Geometry: final body of the model. Coordinates: model frame, mm. A direction names the side the tool comes from. Coordinates: 2 decimals unless noted, no trailing zeros. Write each loop counter-clockwise with the first axis right and the second up, starting at its lowest first coordinate (ties: lowest second). Pieces come first, ordered by that corner, then holes.
from build123d import *

# Parameters (mm, degrees)
ESQUISSE1_W             = 10
ESQUISSE1_H             = 10
BOSS_EXTRU_1_DEPTH      = 10
CONG_1_R                = 10
CONG_2_R                = 3
ESQUISSE2_R             = 1.8
ENL_V_MAT_EXTRU_1_DEPTH = 5
ESQUISSE3_R             = 1.8
ENL_V_MAT_EXTRU_2_DEPTH = 10
CONG_3_R                = 3


with BuildPart() as part:
    # Esquisse1 → Boss.-Extru.1 (new body)
    with BuildSketch(Plane.XY):
        Polygon((5, 29), (0, 29), (0, 0), (5, 0), (5, 14), (32.7, 14), (32.7, 6.5), (52.7, 6.5), (52.7, 14), (55.2, 14), (55.2, 0), (60.2, 0), (60.2, 29), (55.2, 29), (55.2, 21.5), (52.7, 21.5), (52.7, 26.5), (32.7, 26.5), (32.7, 21.5), (5, 21.5), align=None)
        with Locations((42.7, 16.5)):
            Rectangle(ESQUISSE1_W, ESQUISSE1_H, mode=Mode.SUBTRACT)
    extrude(amount=BOSS_EXTRU_1_DEPTH)

    # Congé1
    # the kernel refuses this fillet: 10 mm, written as the material it takes off along each edge
    with BuildSketch(Plane(origin=(52.7, 6.5, -24.206145914), x_dir=(-1, 0, 0), z_dir=(0, 0, 1))) as cong_1_piece_1:
        with BuildLine():
            CenterArc((9.682458366, -10), CONG_1_R, 90, 75.522487814)
            Line((0, -7.5), (-0.193649167, -7.45))
            ThreePointArc((-0.193649167, -7.45), (-0.2, -3.75), (-0.2, 0))
            Line((-0.2, 0), (0, 0.2))
            Line((0, 0.2), (9.682458366, 0.2))
            Line((9.682458366, 0.2), (9.682458366, 0))
        make_face()
    extrude(amount=58.412291828, mode=Mode.SUBTRACT)
    with BuildSketch(Plane(origin=(32.7, 6.5, -24.206145914), x_dir=(0, 1, 0), z_dir=(0, 0, 1))) as cong_1_piece_2:
        with BuildLine():
            CenterArc((10, -9.682458366), CONG_1_R, 104.477512186, 75.522487814)
            Line((0, -9.682458366), (-0.2, -9.682458366))
            Line((-0.2, -9.682458366), (-0.2, 0))
            Line((-0.2, 0), (0, 0.2))
            ThreePointArc((0, 0.2), (3.75, 0.2), (7.45, 0.193649167))
            Line((7.45, 0.193649167), (7.5, 0))
        make_face()
    extrude(amount=58.412291828, mode=Mode.SUBTRACT)
    with BuildSketch(Plane(origin=(52.7, 26.5, -21.650635095), x_dir=(0, -1, 0), z_dir=(0, 0, 1))) as cong_1_piece_3:
        with BuildLine():
            CenterArc((10, -8.660254038), CONG_1_R, 120, 60)
            Line((0, -8.660254038), (-0.2, -8.660254038))
            Line((-0.2, -8.660254038), (-0.2, 0))
            Line((-0.2, 0), (0, 0.2))
            ThreePointArc((0, 0.2), (2.5, 0.2), (4.9, 0.173205081))
            Line((4.9, 0.173205081), (5, 0))
        make_face()
    extrude(amount=53.301270189, mode=Mode.SUBTRACT)
    with BuildSketch(Plane(origin=(32.7, 26.5, -21.650635095), x_dir=(1, 0, 0), z_dir=(0, 0, 1))) as cong_1_piece_4:
        with BuildLine():
            CenterArc((8.660254038, -10), CONG_1_R, 90, 60)
            Line((0, -5), (-0.173205081, -4.9))
            ThreePointArc((-0.173205081, -4.9), (-0.2, -2.5), (-0.2, 0))
            Line((-0.2, 0), (0, 0.2))
            Line((0, 0.2), (8.660254038, 0.2))
            Line((8.660254038, 0.2), (8.660254038, 0))
        make_face()
    extrude(amount=53.301270189, mode=Mode.SUBTRACT)

    # Congé2
    cong_2_edges = [part.edges().sort_by_distance(p)[0] for p in [
        (47.7, 21.5, 5),
        (37.7, 21.5, 5),
        (37.7, 11.5, 5),
        (47.7, 11.5, 5),
    ]]
    fillet(cong_2_edges, radius=CONG_2_R)

    # Esquisse2 → Enlèv. mat.-Extru.1 (cut)
    with BuildSketch(Plane(origin=(60.2, 0, 0), x_dir=(0, 0, -1), z_dir=(1, 0, 0))):
        with Locations(Location((-5, 24, 0), (0, 0, 90))):
            Circle(ESQUISSE2_R)
        with Locations(Location((-5, 4, 0), (0, 0, 90))):
            Circle(ESQUISSE2_R)
    extrude(amount=-ENL_V_MAT_EXTRU_1_DEPTH, mode=Mode.SUBTRACT)

    # Esquisse3 → Enlèv. mat.-Extru.2 (cut)
    with BuildSketch(Plane.ZY):
        with Locations(Location((5, 25, 0), (0, 0, 270))):
            Circle(ESQUISSE3_R)
        with Locations(Location((5, 5, 0), (0, 0, 270))):
            Circle(ESQUISSE3_R)
    extrude(amount=-ENL_V_MAT_EXTRU_2_DEPTH, mode=Mode.SUBTRACT)

    # Congé3
    cong_3_edges = [part.edges().sort_by_distance(p)[0] for p in [
        (53.95, 14, 10),
        (57.7, 0, 10),
        (18.85, 14, 0),
        (2.5, 0, 0),
        (2.5, 29, 0),
        (57.7, 29, 10),
        (18.85, 21.5, 0),
        (53.95, 21.5, 0),
        (57.7, 29, 0),
        (57.7, 0, 0),
        (53.95, 14, 0),
        (53.95, 21.5, 10),
        (18.85, 21.5, 10),
        (2.5, 29, 10),
        (42.7, 6.5, 0),
        (42.7, 26.5, 0),
        (36.360254038, 25.160254038, 0),
        (49.039745962, 25.160254038, 0),
        (2.5, 0, 10),
        (36.258734009, 8.59430585, 0),
        (49.141265991, 8.59430585, 0),
        (42.7, 6.5, 10),
        (42.7, 26.5, 10),
        (36.360254038, 25.160254038, 10),
        (49.039745962, 25.160254038, 10),
        (36.258734009, 8.59430585, 10),
        (18.85, 14, 10),
        (49.141265991, 8.59430585, 10),
    ]]
    fillet(cong_3_edges, radius=CONG_3_R)


solid = part.part
Item 1: Pin query (flat end, axial travel): pin 1 (3 mm diameter, centred on x = 21.5, z = 6, fed in from -Y); pin 2 (5 mm diameter, centred on x = 20, z = 5, fed in from +Y); pin 3 (3 mm diameter, centred on x = 53.5, z = 4.5, fed in from +Y). Return the tip coordinate at first contact, or that it passes through.
Derived:
pin 1: stops at y = 14
pin 2: stops at y = 21.5
pin 3: stops at y = 22.55
Item 2: Pull-direction query (Z, two-part tool) for faces 6 (the cylindrical face through (2.465, 4.169, 3.403)), 7 (the cylindrical face through (57.74, 0.9, 0.86)), 8 (the cylindrical face through (36.424, 25.197, 4.972)); classes: released by +Z, released by -Z, zero draft, split by the parting line, or undercut.
Derived:
face 6: undercut
face 7: released by -Z
face 8: zero draft
Item 3: Section C-C, the plane y = 4. Output: boundary loops of the cut face in (x, z).
Derived:
outline: (0, 0) - (5, 0) - (5, 3.5) - (0, 3.5) - close; (0, 6.5) - (5, 6.5) - (5, 10) - (0, 10) - close; (55.2, 0) - (60.2, 0) - (60.2, 3.2) - (55.2, 3.2) - close; (55.2, 6.8) - (60.2, 6.8) - (60.2, 10) - (55.2, 10) - close
Item 4: Section A-A, the plane x = 31. Output: boundary loops of the cut face in (y, z).
Derived:
outline: (14, 3) arc R3 ccw to (17, 0) - (18.5, 0) arc R3 ccw to (21.5, 3) - (21.5, 7) arc R3 ccw to (18.5, 10) - (17, 10) arc R3 ccw to (14, 7) - close
Item 5: Material intervals for probe 1 along Z at (x, y) = (57.4, 24); probe 2 along X at (y, z) = (26.75, 3.25); probe 3 along X at (y, z) = (10.75, 2), sorted ascending.
Derived:
probe 1: z = 0 to 3.2, 6.8 to 10
probe 2: x = 0 to 5, 55.2 to 60.2
probe 3: x = 0 to 5, 34.41 to 50.99, 55.2 to 60.2
Item 6: Set-up query: faces 1 (the cylindrical face through (42.68, 25.64, 9.1)), 2 (the flat face through (58, 29, 5)), 3 (the flat face through (43, 11.5, 5)), 4 (the cylindrical face through (57.735, 4.831, 3.403)), 5 (the cylindrical face through (42.68, 25.6, 0.86)). Return all of +Z, -Z, +X, -X, +Y, -Y with unobstructed straight access to the full face (end or side cutting, diameter ignored); none if empty.
Derived:
face 1: +Z, +Y
face 2: +Z, -Z, +X, -X, +Y
face 3: +Z, -Z
face 4: +X
face 5: -Z, +Y
Item 7: Section B-B, the plane z = 5. State how many separate pieces and enclosed holes the cut face has, plus the area to 3 significant figures.
Derived:
separate pieces: 5
enclosed holes: 1
area: 689 mm2
Item 8: Section D-D, the plane z = 1.25. Output: boundary loops of the cut face in (x, y), plus the area to 3 significant figures.
Derived:
outline: (0, 0.56) - (5, 0.56) - (5, 14.56) - (33.15, 14.56) arc R9.44 ccw to (42.38, 7.06) - (43.02, 7.06) arc R9.44 ccw to (52.25, 14.56) - (55.2, 14.56) - (55.2, 0.56) - (60.2, 0.56) - (60.2, 28.44) - (55.2, 28.44) - (55.2, 20.94) - (52.37, 20.94) arc R9.44 ccw to (44.04, 25.94) - (41.36, 25.94) arc R9.44 ccw to (33.03, 20.94) - (5, 20.94) - (5, 28.44) - (0, 28.44) - close; hole (37.7, 14.5) arc R3 ccw to (40.7, 11.5) - (44.7, 11.5) arc R3 ccw to (47.7, 14.5) - (47.7, 18.5) arc R3 ccw to (44.7, 21.5) - (40.7, 21.5) arc R3 ccw to (37.7, 18.5) - close
area: 687 mm2
